Autodesk Inventor part; units mm, degrees
ref_plane "YZ Plane" through (0, 0, 0) normal (1, 0, 0) x (0, 1, 0)
ref_plane "XZ Plane" through (0, 0, 0) normal (0, 1, 0) x (-1, 0, 0)
ref_plane "XY Plane" through (0, 0, 0) normal (0, 0, 1) x (1, 0, 0)
sketch "Sketch1" plane through (0, 0, 0) normal (0, 1, 0) x (-1, 0, 0)
  line L0 (0, 0) -> (-50, 0)
  line L1 (-50, 0) -> (-50, -50)
  line L2 (-50, -50) -> (0, -50)
  line L3 (0, -50) -> (0, 0)
  line L4 (0, 0) -> (-1500, 0)
  line L5 (-1500, 0) -> (-1500, -700)
  line L6 (-1500, -700) -> (0, -700)
  line L7 (0, -700) -> (0, 0)
  line L8 (0, -700) -> (-50, -700)
  line L9 (-50, -700) -> (-50, -650)
  line L10 (-50, -650) -> (0, -650)
  line L11 (0, -650) -> (0, -700)
  line L12 (-1500, -700) -> (-1450, -700)
  line L13 (-1450, -700) -> (-1450, -650)
  line L14 (-1450, -650) -> (-1500, -650)
  line L15 (-1500, -650) -> (-1500, -700)
  line L16 (-1500, 0) -> (-1450, 0)
  line L17 (-1450, 0) -> (-1450, -50)
  line L18 (-1450, -50) -> (-1500, -50)
  line L19 (-1500, -50) -> (-1500, 0)
  point P0 (-1500, -50)
  point P1 (-1450, 0)
  point P2 (0, -650)
  dimension "d0" = 50
  dimension "d1" = 50
  dimension "d2" = 1500
  dimension "d3" = 700
  dimension "d4" = 50
  dimension "d5" = 50
  dimension "d6" = 50
  dimension "d7" = 50
  dimension "d8" = 50
  dimension "d9" = 50
extrude "Extrusion1" add sketch "Sketch1" along normal blind 330 contours L3 L2 L1 L0 | L17 L18 L5 L4 | L7 L6 L9 L10 | L14 L13 L6 L5
sketch "Sketch2" plane through (0, 330, 0) normal (0, 1, 0) x (1, 0, 0)
  line L0 (50, 700) -> (0, 700)
  line L1 (0, 700) -> (1500, 700)
  line L2 (1500, 700) -> (1500, 0)
  line L3 (1500, 0) -> (0, 0)
  line L4 (0, 0) -> (0, 700)
chamfer "Chamfer1" distance 10 angle 45 16 edges at (0, 165, -650) (50, 165, -650) (50, 165, -700) (0, 165, -700) (1450, 165, -650) (1450, 165, -700) (1500, 165, -700) (1500, 165, -650) (1450, 165, 0) (1500, 165, -50) (1500, 165, 0) (1450, 165, -50) (0, 165, -50) (0, 165, 0) (50, 165, 0) (50, 165, -50)
extrude "Extrusion2" add sketch "Sketch2" along normal blind 20
sketch "Sketch3" plane through (0, 330, 0) normal (0, -1, 0) x (1, 0, 0)
  line L0 (50, -10) -> (50, -40)
  line L1 (1450, -40) -> (1450, -10)
  line L2 (50, -10) -> (1450, -10)
  line L3 (1450, -10) -> (1450, -40)
  line L4 (1450, -40) -> (50, -40)
  line L5 (50, -40) -> (50, -10)
  line L6 (1490, -50) -> (1460, -50)
  line L7 (1460, -650) -> (1490, -650)
  line L8 (1460, -50) -> (1490, -50)
  line L9 (1490, -50) -> (1490, -650)
  line L10 (1490, -650) -> (1460, -650)
  line L11 (1460, -650) -> (1460, -50)
  line L12 (50, -660) -> (1450, -660)
  line L13 (1450, -660) -> (1450, -690)
  line L14 (1450, -690) -> (50, -690)
  line L15 (50, -690) -> (50, -660)
  line L16 (40, -50) -> (10, -50)
  line L17 (10, -50) -> (40, -50)
  line L18 (40, -50) -> (40, -650)
  line L19 (40, -650) -> (10, -650)
  line L20 (10, -650) -> (10, -50)
  point P0 (0, 0)
extrude "Extrusion3" add sketch "Sketch3" along normal blind 50
properties part number "Table"
Geometry check sheet. Reference: the model listing, model coordinates, mm. A direction names the side the tool comes from. Round coordinates to 2 decimals unless told otherwise and drop trailing zeros. Order: outer loops, then holes, each group sorted by start corner. A loop starts at its lowest first (then second) coordinate and runs counter-clockwise, first axis right, second up. Notation, with made-up numbers: M 60,80 L 95,80 A14 ccw 95,97 Z; hole C -19.75,29.25 d8. An arc over 180 degrees is marked long. Answer in a Markdown table with one row per item. Add a question column.
Item 1: Sectioned sample at B-B, the plane x = 466. Enter the section's corners in (y, z).
Item 2: Draft check along X on faces 1 (the face through (1475, 0, -25)), 2 (the face through (1490, 305, -346)), 3 (the face through (50, 138, -25)). Enter one of: released by +X, released by -X, zero draft, split by the parting line, or undercut.
Item 3: Material ranges on L1, parallel to X at y = 308.5, z = -468.5; L2, parallel to Y at x = 509.5, z = -275.5, recorded low to high. Write a range as [from, to].
Item 4: Sectioned sample at C-C, the plane z = -403. Enter the section's corners in (x, y), plus the area to 3 significant figures.
Item 5: Sectioned sample at A-A, the plane y = 77.5. State how many separate pieces and enclosed holes the cut face has, plus the area to 3 significant figures.
Item 6: Depth check by flat-ended pin: pin 1 Ø3 at (x, z) = (3, -694) entering from -Y; pin 2 Ø25 at (x, y) = (615, 312.5) entering from -Z; pin 3 Ø2 at (y, z) = (307.5, -540) entering from +X; pin 4 Ø24 at (x, z) = (30, -294.5) entering from -Y. Enter the tip coordinate at first touch or a pass-through.
Item 7: Set-up check for faces 4 (the face through (40, 305, -346)), 5 (the face through (740, 305, -10)), 6 (the face through (740, 280, -25)), 7 (the face through (25, 138, -650)): record each of +Z, -Z, +X, -X, +Y, -Y from which the full face is reachable in a straight line by a thin tool's end or side.
Filled in:
| question | item | result |
|---|---|---|
| 1 | outline | M 280,-690 L 330,-690 L 330,-700 L 350,-700 L 350,0 L 330,0 L 330,-10 L 280,-10 L 280,-40 L 330,-40 L 330,-660 L 280,-660 Z |
| 2 | face 1 | zero draft |
| 2 | face 2 | released by +X |
| 2 | face 3 | undercut |
| 3 | L1 | x = [10, 40], [1460, 1490] |
| 3 | L2 | y = [330, 350] |
| 4 | outline | M 0,330 L 10,330 L 10,280 L 40,280 L 40,330 L 1460,330 L 1460,280 L 1490,280 L 1490,330 L 1500,330 L 1500,350 L 0,350 Z |
| 4 | area | 33,000 mm² |
| 5 | separate pieces | 4 |
| 5 | enclosed holes | 0 |
| 5 | area | 9,200 mm² |
| 6 | pin 1 | stops at y = 0 |
| 6 | pin 2 | stops at z = -690 |
| 6 | pin 3 | stops at x = 1490 |
| 6 | pin 4 | stops at y = 280 |
| 7 | face 4 | -Y |
| 7 | face 5 | +Z, -Y |
| 7 | face 6 | +Z, -Z, -Y |
| 7 | face 7 | +X, -X, -Y |
